Check sheet for the modelled part. Datum: model origin and axes. Units: mm. A direction names the side the tool comes from. Round coordinates to 2 decimals unless told otherwise and drop trailing zeros. Loops run counter-clockwise (first coordinate to the right, second up) from the corner with the lowest first, then second, coordinate; pieces in that order, holes last. Notation, with made-up numbers: (62.25, 44) - (82.25, 44) arc R13 cw to (82.25, 52) - close; hole circle Ø11 at (-10, -20). An arc over 180 degrees is marked (long way). Answer in a Markdown table with one row per item. Add a question column.
(1) Access from +Z, -Z, +X, -X, +Y, -Y to the whole of each face (thin tool, end or side, straight path). Record for faces 1 (the cylindrical face through (10.18, -6.26, -10.77)), 2 (the cylindrical face through (10.18, 57.06, -14.63)), 3 (the flat face through (13, -12.7, -13)).
(2) Thickness scan on line 1 along Y through (x, z) = (21.5, -148); line 2 along Z through (x, y) = (12.75, -8). Record the ranges inside material, lowest first.
(3) Cross-section at B-B on x = 12.7. Enter the section's corners in (y, z) (3 decimals).
(4) Cross-section at A-A on z = -12.7. Enter the section's corners in (x, y) (3 decimals), then the cut area to 3 significant figures.
(5) Gauge pin test, flat ends, axial feed: pin 1 (3 mm diameter, centred on x = 15, z = -69, fed in from +Y); pin 2 (5 mm diameter, centred on x = 13, z = -100.5, fed in from -Y). Record the tip position at first contact, or that the pin passes through.
(6) Cross-section at C-C on z = -39. Enter the section's corners in (x, y), then the cut area to 3 significant figures.
Autodesk Inventor part; units mm, degrees
ref_plane "YZ Plane" through (0, 0, 0) normal (1, 0, 0) x (0, 1, 0)
ref_plane "XZ Plane" through (0, 0, 0) normal (0, 1, 0) x (-1, 0, 0)
ref_plane "XY Plane" through (0, 0, 0) normal (0, 0, 1) x (1, 0, 0)
sketch "Sketch1" plane through (0, 0, 0) normal (1, 0, 0) x (0, 1, 0)
  line L0 (0, 0) -> (50.8, 0)
  line L1 (50.8, 0) -> (50.8, -203.2)
  line L2 (50.8, -203.2) -> (0, -203.2)
  line L3 (0, -203.2) -> (0, 0)
  dimension "d0" = 50.8
  dimension "d1" = 203.2
extrude "Extrusion1" add sketch "Sketch1" along normal blind 25.4
sketch "Sketch2" plane through (0, 50.8, 0) normal (0, 1, 0) x (1, 0, 0)
  circle A0 centre (12.7, 12.7) radius 3.175
  line L0 (0, 0) -> (0, 203.2)
  line L1 (0, 0) -> (25.4, 0)
  line L2 (25.4, 203.2) -> (25.4, 0)
  line L3 (0, 203.2) -> (25.4, 203.2)
  point P0 (0, 0)
  dimension "d4" = 6.35
  dimension "d5" = 12.7
  dimension "d6" = 12.7
extrude "Extrusion2" add sketch "Sketch2" along normal blind 12.7 contours A0
sketch "Sketch3" plane through (0, 0, -203.2) normal (0, -1, 0) x (1, 0, 0)
  line L0 (0, 0) -> (0, 203.2)
  line L1 (0, 0) -> (25.4, 0)
  line L2 (25.4, 203.2) -> (25.4, 0)
  line L3 (0, 203.2) -> (25.4, 203.2)
  circle A0 centre (12.7, 190.5) radius 3.175
  dimension "d9" = 6.35
  dimension "d10" = 12.7
  dimension "d11" = 12.7
extrude "Extrusion3" add sketch "Sketch3" along normal blind 12.7 contours A0
properties part number "StressArm"
Answers:
| question | item | result |
|---|---|---|
| 1 | face 1 | -Y |
| 1 | face 2 | +Y |
| 1 | face 3 | +Z, -Z, +X, -X, -Y |
| 2 | line 1 | y = 0 to 50.8 |
| 2 | line 2 | z = -15.87 to -9.53 |
| 3 | outline | (-12.7, -15.875) - (0, -15.875) - (0, -203.2) - (50.8, -203.2) - (50.8, -15.875) - (63.5, -15.875) - (63.5, -9.525) - (50.8, -9.525) - (50.8, 0) - (0, 0) - (0, -9.525) - (-12.7, -9.525) - close |
| 4 | outline | (0, 0) - (9.525, 0) - (9.525, -12.7) - (15.875, -12.7) - (15.875, 0) - (25.4, 0) - (25.4, 50.8) - (15.875, 50.8) - (15.875, 63.5) - (9.525, 63.5) - (9.525, 50.8) - (0, 50.8) - close |
| 4 | area | 1,450 mm^2 |
| 5 | pin 1 | stops at y = 50.8 |
| 5 | pin 2 | stops at y = 0 |
| 6 | outline | (0, 0) - (25.4, 0) - (25.4, 50.8) - (0, 50.8) - close |
| 6 | area | 1,290 mm^2 |
